The drawing under review shows one solid part. Ordinate dimensions are in mm from its lowest x, y, z. A direction names the side the tool comes from. Round coordinates to 2 decimals unless told otherwise and drop trailing zeros. Write each loop counter-clockwise with the first axis right and the second up, starting at its lowest first coordinate (ties: lowest second). Pieces come first, ordered by that corner, then holes. Notation, with made-up numbers: (1, 35.25) - (48, 35.25) arc R17 cw to (48, 46.25) - close; hole circle Ø5 at (-25, 46). An arc over 180 degrees is marked (long way). One line per question, with ' | ' between items. Start each with the question number.
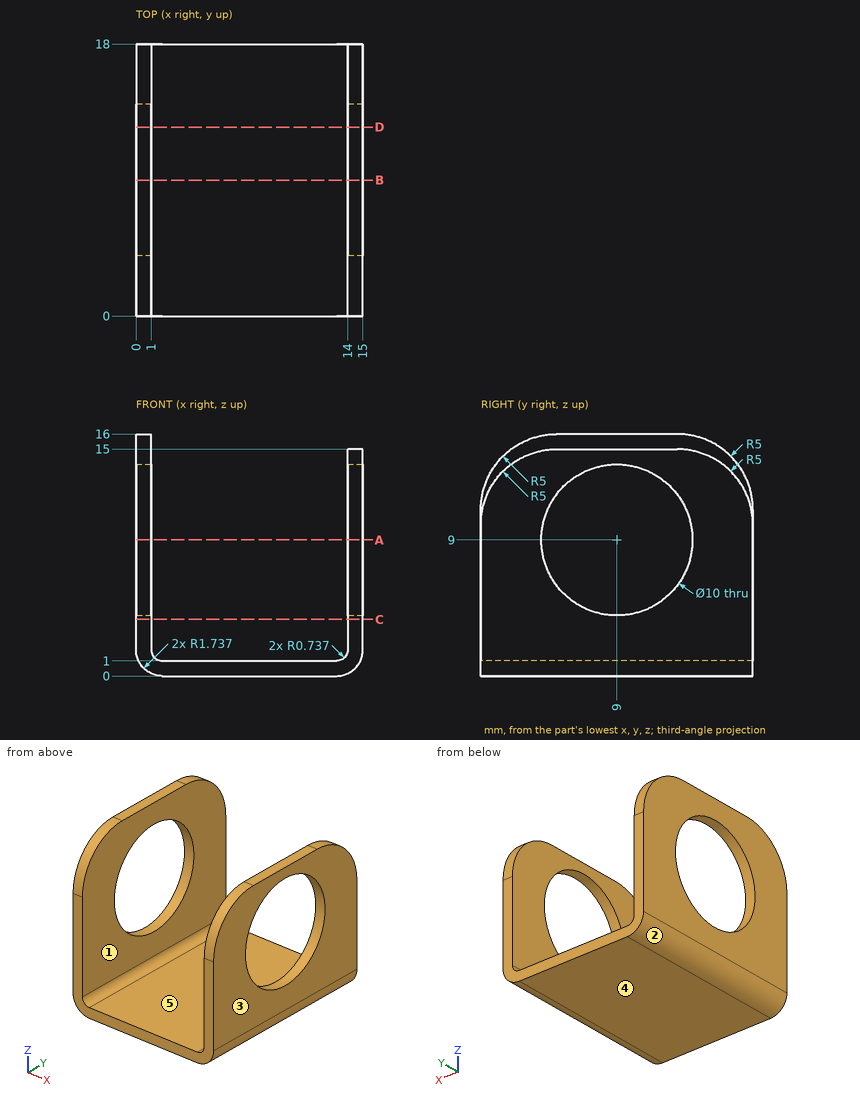
1. Wall thickness on line 1 along X through (y, z) = (13, 1.75); line 2 along Z through (x, y) = (1.75, 2.75); line 3 along Y through (x, z) = (14.5, 4.5): over which ranges is each line inside the solid? List them lowest first. Write a range as [from, to].
2. Add section B-B, the plane y = 9. Write out the cut boundary in (x, z).
3. Machinability: for the marked faces 4 and 5, which of the approach directions +Z, -Z, +X, -X, +Y, -Y give a long, thin tool a straight path to every point of the face, cutting with its end or side? Answer none if there is none.
4. Add section D-D, the plane y = 12.5. Write out the cut boundary in (x, z).
5. Add section C-C, the plane z = 3.75. Write out the cut boundary in (x, y).
6. The part is to be moulded in two halves that separate along X. For the marked faces 1, 2 and 3, say which applies: pulls with the +X half, pulls with the -X half, needs draft (parallel to the pull), parting line crosses it, or undercut.
7. Clearance check with flat-ended pins moving along their axes: P1, Ø4, axis at x = 9.5, y = 15.5, coming from the +Z side; P2, Ø4, axis at y = 6, z = 9.5, coming from the -X side; P3, Ø1.5, axis at x = 13, y = 14, coming from the +Z side (1 decimal); P4, Ø0.5, axis at x = 14.5, y = 11, coming from the +Z side. State where each tip first meets the part, or that it passes through.
8. Add section A-A, the plane z = 9. Write out the cut boundary in (x, y), then the cut area to 3 significant figures.
Geometry check:
1) line 1: x = [0, 1], [14, 15] | line 2: z = [0, 1] | line 3: y = [0, 6.82], [11.18, 18]
2) outline: (0, 1.74) arc R1.74 ccw to (1.74, 0) - (13.26, 0) arc R1.74 ccw to (15, 1.74) - (15, 4) - (14, 4) - (14, 1.74) arc R0.74 cw to (13.26, 1) - (1.74, 1) arc R0.74 cw to (1, 1.74) - (1, 4) - (0, 4) - close; (0, 14) - (1, 14) - (1, 16) - (0, 16) - close; (14, 14) - (15, 14) - (15, 15) - (14, 15) - close
3) face 4: -Z, +X, -X, +Y, -Y | face 5: +Z, +Y, -Y
4) outline: (0, 1.74) arc R1.74 ccw to (1.74, 0) - (13.26, 0) arc R1.74 ccw to (15, 1.74) - (15, 5.43) - (14, 5.43) - (14, 1.74) arc R0.74 cw to (13.26, 1) - (1.74, 1) arc R0.74 cw to (1, 1.74) - (1, 5.43) - (0, 5.43) - close; (0, 12.57) - (1, 12.57) - (1, 16) - (0, 16) - close; (14, 12.57) - (15, 12.57) - (15, 15) - (14, 15) - close
5) outline: (0, 0) - (1, 0) - (1, 18) - (0, 18) - close; (14, 0) - (15, 0) - (15, 18) - (14, 18) - close
6) face 1: undercut | face 2: pulls with the -X half | face 3: pulls with the +X half
7) P1: stops at z = 1 | P2: stops at x = 0 | P3: stops at z = 1.2 | P4: stops at z = 15
8) outline: (0, 0) - (1, 0) - (1, 4) - (0, 4) - close; (0, 14) - (1, 14) - (1, 18) - (0, 18) - close; (14, 0) - (15, 0) - (15, 4) - (14, 4) - close; (14, 14) - (15, 14) - (15, 18) - (14, 18) - close | area: 16.0 mm2
